Build history of the part. All positions in model axes, mm. Give positions to 0.01 mm unless a question says otherwise; leave off trailing zeros. Order: outer loops, then holes, each group sorted by start corner. A loop starts at its lowest first (then second) coordinate and runs counter-clockwise, first axis right, second up. Notation, with made-up numbers: (45, -18.75) - (70, -18.75) arc R22 ccw to (70, 2.25) - close; hole circle Ø7 at (75, 52.25). An arc over 180 degrees is marked (long way). Write each question's results on one line, items separated by ' | '. Start each with the question number.
1) Cut at A-A on x = 8.5. List the corners of the cut face in (y, z), plus the area to 4 significant figures.
2) Cut at C-C on z = -25.5. List the corners of the cut face in (x, y), plus the area to 4 significant figures.
3) Drill centre lines: line 1 along Z through (x, y) = (7, 1.6); line 2 along X through (y, z) = (0.3, -32.5). Where is each one in solid material? Low to high. Write a range as from..to.
4) Cut at B-B on y = 0.7. List the corners of the cut face in (x, z).
from build123d import *

# Parameters (mm, degrees)
SKETCH1_W           = 119
SKETCH1_H           = 103
BOSS_EXTRUDE1_DEPTH = 2.5
SKETCH3_W           = 55
SKETCH3_H           = 44
CUT_EXTRUDE2_DEPTH  = 10
SKETCH4_W           = 103
SKETCH4_H           = 2.5
BOSS_EXTRUDE2_DEPTH = 1.5
SKETCH5_W           = 103
SKETCH5_H           = 2.5
BOSS_EXTRUDE3_DEPTH = 1.5


with BuildPart() as part:
    # Sketch1 → Boss-Extrude1 (new body)
    with BuildSketch(Plane(origin=(0, 0, 0), x_dir=(1, 0, 0), z_dir=(0, 1, 0))):
        Rectangle(SKETCH1_W, SKETCH1_H)
    extrude(amount=BOSS_EXTRUDE1_DEPTH)

    # Sketch3 → Cut-Extrude2 (cut)
    with BuildSketch(Plane(origin=(0, 2.5, 0), x_dir=(1, 0, 0), z_dir=(0, 1, 0))):
        with Locations((9, 16.5)):
            Rectangle(SKETCH3_W, SKETCH3_H)
    extrude(amount=-CUT_EXTRUDE2_DEPTH, mode=Mode.SUBTRACT)

    # Sketch4 → Boss-Extrude2 (add)
    with BuildSketch(Plane.ZY.offset(59.5)):
        with Locations((0, 1.25)):
            Rectangle(SKETCH4_W, SKETCH4_H)
    extrude(amount=BOSS_EXTRUDE2_DEPTH)

    # Sketch5 → Boss-Extrude3 (add)
    with BuildSketch(Plane(origin=(59.5, 0, 0), x_dir=(0, 0, -1), z_dir=(1, 0, 0))):
        with Locations((0, 1.25)):
            Rectangle(SKETCH5_W, SKETCH5_H)
    extrude(amount=BOSS_EXTRUDE3_DEPTH)


solid = part.part
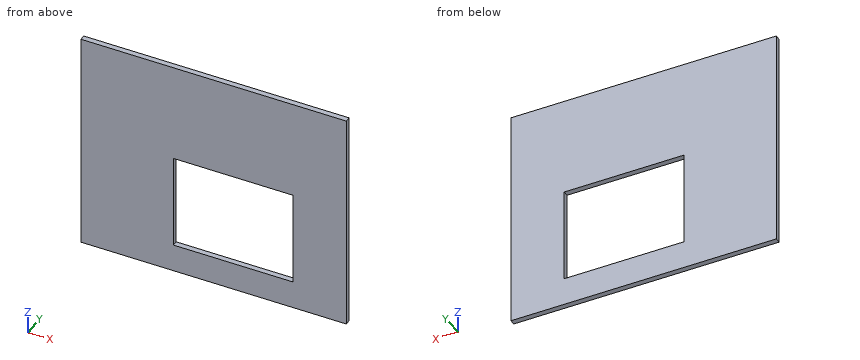
Results:
1) outline: (0, -51.5) - (2.5, -51.5) - (2.5, -38.5) - (0, -38.5) - close; (0, 5.5) - (2.5, 5.5) - (2.5, 51.5) - (0, 51.5) - close | area: 147.5 mm^2
2) outline: (-61, 0) - (-18.5, 0) - (-18.5, 2.5) - (-61, 2.5) - close; (36.5, 0) - (61, 0) - (61, 2.5) - (36.5, 2.5) - close | area: 167.5 mm^2
3) line 1: -51.5..-38.5, 5.5..51.5 | line 2: -61..-18.5, 36.5..61
4) outline: (-61, -51.5) - (61, -51.5) - (61, 51.5) - (-61, 51.5) - close; hole (-18.5, -38.5) - (36.5, -38.5) - (36.5, 5.5) - (-18.5, 5.5) - close
